The listing builds one solid part. Answer for the finished solid, in the listing's coordinates (mm). Face numbers are marked on the shaded views. A direction names the side the tool comes from. Give positions to 0.01 mm unless a question says otherwise; leave off trailing zeros. Loops run counter-clockwise (first coordinate to the right, second up) from the corner with the lowest first, then second, coordinate; pieces in that order, holes last. Notation, with made-up numbers: (79.5, -18.75) - (86.5, -18.75) arc R22 cw to (86.5, 15.25) - close; hole circle Ø8 at (41.25, 3). An arc over 180 degrees is marked (long way). Write each question's results on one line, items separated by ' | '.
from build123d import *

# Parameters (mm, degrees)
BOSS_EXTRUDE1_DEPTH     = 7.5
SKETCH4_R               = 4.1
CUT_EXTRUDE1_DEPTH      = 10
SKETCH5_R               = 1.5
CUT_EXTRUDE2_DEPTH      = 5
CUT_EXTRUDE4_REACH      = 40.591
CUT_EXTRUDE4_END_RADIUS = 4.1
SKETCH7_R               = 1.5
BOSS_EXTRUDE2_DEPTH     = 20
CUT_EXTRUDE5_DEPTH      = 20
CUT_EXTRUDE6_DEPTH      = 8
SKETCH13_R              = 1.5
CUT_EXTRUDE7_DEPTH      = 16
SKETCH14_R              = 1.5
CUT_EXTRUDE8_DEPTH      = 4
CUT_EXTRUDE9_START      = -1
CUT_EXTRUDE9_DEPTH      = 2.6
SKETCH16_W              = 3
SKETCH16_H              = 13
CUT_EXTRUDE10_DEPTH     = 36.128336141
FILLET1_R               = 8


with BuildPart() as part:
    # Sketch2 → Boss-Extrude1 (new, symmetric)
    with BuildSketch(Plane(origin=(0, 0, 0), x_dir=(1, 0, 0), z_dir=(0, 1, 0))):
        Polygon((-16, -8), (-16, 8), (0, 8), (16, 6.5), (21, 6.5), (21, -6.5), (16, -6.5), (0, -8), align=None)
    extrude(amount=BOSS_EXTRUDE1_DEPTH, both=True)

    # Sketch4 → Cut-Extrude1 (cut)
    with BuildSketch(Plane(origin=(0, 7.5, 0), x_dir=(1, 0, 0), z_dir=(0, 1, 0))):
        with Locations(Location((-7.259972257, 0, 0), (0, 0, 270))):
            Circle(SKETCH4_R)
    extrude(amount=-CUT_EXTRUDE1_DEPTH, mode=Mode.SUBTRACT)

    # Sketch5 → Cut-Extrude2 (cut)
    with BuildSketch(Plane(origin=(0, -2.5, 0), x_dir=(1, 0, 0), z_dir=(0, 1, 0))):
        with Locations(Location((-7.259972257, 0, 0), (0, 0, 270))):
            Circle(SKETCH5_R)
    extrude(amount=-CUT_EXTRUDE2_DEPTH, mode=Mode.SUBTRACT)

    # Cut-Extrude4: up to this cylinder (the profile starts outside it)
    cut_extrude4_end = Plane(origin=(-7.259972257, 2.5, 0), z_dir=(0, 1, 0)) * Cylinder(CUT_EXTRUDE4_END_RADIUS, 90.382, mode=Mode.PRIVATE)
    # Sketch7 → Cut-Extrude4 (cut, up to the surface)
    with BuildSketch(Plane.ZY.offset(16), mode=Mode.PRIVATE) as cut_extrude4_sk1:
        with Locations((0, 2.5)):
            Circle(SKETCH7_R)
    cut_extrude4_tool1 = extrude(cut_extrude4_sk1.sketch, amount=-CUT_EXTRUDE4_REACH, mode=Mode.PRIVATE) - cut_extrude4_end
    add(cut_extrude4_tool1.solids().sort_by_distance((-16, 2.5, 0))[0], mode=Mode.SUBTRACT)

    # Sketch8 → Boss-Extrude2 (add)
    with BuildSketch(Plane(origin=(0, 7.5, 0), x_dir=(1, 0, 0), z_dir=(0, 1, 0))):
        Polygon((7, 7.34375), (7, -7.34375), (16, -6.5), (21, -6.5), (21, 6.5), (16, 6.5), align=None)
    extrude(amount=BOSS_EXTRUDE2_DEPTH)

    # Sketch11 → Cut-Extrude5 (cut)
    with BuildSketch(Plane(origin=(0, 27.5, 0), x_dir=(1, 0, 0), z_dir=(0, 1, 0))):
        Polygon((11, 6.96875), (11, -6.96875), (14, -6.6875), (14, 6.6875), align=None)
    extrude(amount=-CUT_EXTRUDE5_DEPTH, mode=Mode.SUBTRACT)

    # Sketch12 → Cut-Extrude6 (cut)
    with BuildSketch(Plane(origin=(0, 27.5, 0), x_dir=(1, 0, 0), z_dir=(0, 1, 0))):
        Polygon((14, 6.6875), (14, -6.6875), (16, -6.5), (21, -6.5), (21, 6.5), (16, 6.5), align=None)
    extrude(amount=-CUT_EXTRUDE6_DEPTH, mode=Mode.SUBTRACT)

    # Sketch13 → Cut-Extrude7 (cut)
    with BuildSketch(Plane(origin=(21, 0, 0), x_dir=(0, 0, -1), z_dir=(1, 0, 0))):
        with Locations((-3, 16.5)):
            Circle(SKETCH13_R)
        with Locations((3, 16.5)):
            Circle(SKETCH13_R)
        with Locations((-3.1, 10.5)):
            Circle(SKETCH13_R)
        with Locations((3.1, 10.5)):
            Circle(SKETCH13_R)
    extrude(amount=-CUT_EXTRUDE7_DEPTH, mode=Mode.SUBTRACT)

    # Sketch14 → Cut-Extrude8 (cut)
    with BuildSketch(Plane.ZY.offset(-7)):
        with Locations((-3.5, 22.5)):
            Circle(SKETCH14_R)
        with Locations((3.5, 22.5)):
            Circle(SKETCH14_R)
    extrude(amount=-CUT_EXTRUDE8_DEPTH, mode=Mode.SUBTRACT)

    # Sketch15 → Cut-Extrude9 (cut)
    with BuildSketch(Plane.ZY.offset(-7).offset(CUT_EXTRUDE9_START)):
        Polygon((4.658845727, 13.2), (1.541154273, 13.2), (-0.017691454, 10.5), (1.541154273, 7.8), (4.658845727, 7.8), (6.217691454, 10.5), align=None)
    cut_extrude9 = extrude(amount=CUT_EXTRUDE9_DEPTH, mode=Mode.SUBTRACT)

    # Mirror1: Cut-Extrude9 across plane
    add(cut_extrude9.mirror(Plane.XY), mode=Mode.SUBTRACT)

    # Sketch16 → Cut-Extrude10 (cut, through all)
    with BuildSketch(Plane(origin=(0, 19.5, 0), x_dir=(1, 0, 0), z_dir=(0, 1, 0))):
        with Locations((19.5, 0)):
            Rectangle(SKETCH16_W, SKETCH16_H)
    extrude(amount=-CUT_EXTRUDE10_DEPTH, mode=Mode.SUBTRACT)

    # Fillet1
    fillet1_edges = [part.edges().sort_by_distance(p)[0] for p in [
        (18, -7.5, 0),
    ]]
    fillet(fillet1_edges, radius=FILLET1_R)


solid = part.part
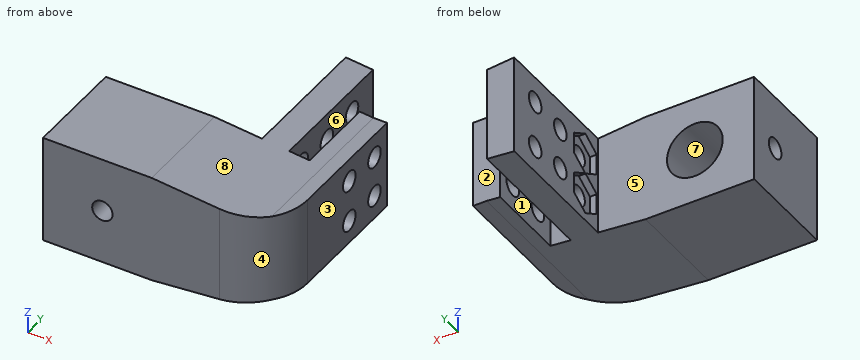
Item 1: Flat-ended cylindrical pins translate along their axes: P1, Ø0.6, axis at x = 16.5, y = 11.5, coming from the -Z side; P2, Ø1.8, axis at y = 10.5, z = -3.1, coming from the -X side; P3, Ø1, axis at x = 3, y = 1.5, coming from the +Z side; P4, Ø4.5, axis at y = 11, z = 1, coming from the -X side. Find the tip coordinate at first contact, or state that the pin passes through.
Values found:
P1: stops at z = -6.5 | P2: passes through | P3: stops at z = 7.77 | P4: stops at x = 7
Item 2: A cutting plane is placed at A-A, the plane y = 16.5. Determine the outline of the cut face in (x, z).
Values found:
outline: (7, -7.34) - (11, -6.97) - (11, -4.5) - (7, -4.5) - close; (7, -1.5) - (11, -1.5) - (11, 1.5) - (7, 1.5) - close; (7, 4.5) - (11, 4.5) - (11, 6.97) - (7, 7.34) - close; (14, -6.69) - (16, -6.5) - (18, -6.5) - (18, -4.5) - (14, -4.5) - close; (14, -1.5) - (18, -1.5) - (18, 1.5) - (14, 1.5) - close; (14, 4.5) - (18, 4.5) - (18, 6.5) - (16, 6.5) - (14, 6.69) - close
Item 3: A cutting plane is placed at B-B, the plane y = 8.5. Determine the outline of the cut face in (x, z).
Values found:
outline: (7, -7.34) - (11, -6.97) - (11, 6.97) - (7, 7.34) - (7, 5.06) - (8, 5.06) - (8, 1.14) - (7, 1.14) - (7, -1.14) - (8, -1.14) - (8, -5.06) - (7, -5.06) - close; (14, -6.69) - (16, -6.5) - (18, -6.5) - (18, 6.5) - (16, 6.5) - (14, 6.69) - close
Item 4: For a pull along Z with two mould halves and no side action, classify the marked faces 6, 7 and 8 as released by +Z, released by -Z, zero draft, split by the parting line, or undercut.
Values found:
face 6: zero draft | face 7: undercut | face 8: released by +Z
Item 5: Find the intervals of material crossed by line 1 along X through (y, z) = (17.5, 5.5); line 2 along X through (y, z) = (8, 4.5); line 3 along Y through (x, z) = (-13.15, 0), in increasing order. Write a range as [from, to].
Values found:
line 1: x = [7, 11], [14, 18] | line 2: x = [8, 11], [14, 18] | line 3: y = [-7.5, 1], [4, 7.5]
Item 6: A cutting plane is placed at D-D, the plane y = 2.5. Determine the outline of the cut face in (x, z), plus the area to 3 significant figures.
Values found:
outline: (-16, -8) - (0, -8) - (16, -6.5) - (18, -6.5) - (18, 6.5) - (16, 6.5) - (0, 8) - (-16, 8) - (-16, 1.5) - (-11.08, 1.5) arc R4.1 cw (long way) to (-11.08, -1.5) - (-16, -1.5) - close | area: 447 mm²
Item 7: For the marked faces 1, 2, 3, 4 and 5, determine the directions among +Z, -Z, +X, -X, +Y, -Y from which every point of the face is accessible in a straight line to the end or side of a thin tool.
Values found:
face 1: +Z, -Z, +Y | face 2: +Z, -Z, +X, +Y | face 3: +Z, -Z, +X, +Y, -Y | face 4: +Z, -Z, +X, -Y | face 5: +Z, -Z, -X, +Y
Item 8: A cutting plane is placed at C-C, the plane z = 1. Determine the outline of the cut face in (x, y).
Values found:
outline: (-16, -7.5) - (-8.38, -7.5) - (-8.38, -2.5) - (-11.24, -2.5) - (-11.24, 1.38) - (-16, 1.38) - close; (-16, 3.62) - (-11.24, 3.62) - (-11.24, 7.5) - (-16, 7.5) - close; (-6.14, -7.5) - (10, -7.5) arc R8 ccw to (18, 0.5) - (18, 19.5) - (14, 19.5) - (14, 7.5) - (11, 7.5) - (11, 27.5) - (7, 27.5) - (7, 12.26) - (8, 12.26) - (8, 8.74) - (7, 8.74) - (7, 7.5) - (-3.28, 7.5) - (-3.28, -2.5) - (-6.14, -2.5) - close
